from build123d import *

# Parameters (mm, degrees)
BOSS_EXTRUDE1_DEPTH = 115
SKETCH4_W           = 110.804791126
SKETCH4_H           = 80.151186243
CUT_EXTRUDE1_DEPTH  = 15
SKETCH6_W           = 33
SKETCH6_H           = 45.5
CUT_EXTRUDE2_DEPTH  = 40
CUT_EXTRUDE3_DEPTH  = 144.740217058
SKETCH10_W          = 47
SKETCH10_H          = 20
SKETCH10_W_2        = 40
BOSS_EXTRUDE2_DEPTH = 15


with BuildPart() as part:
    # Sketch3 → Boss-Extrude1 (new body)
    with BuildSketch(Plane(origin=(0, 0, 0), x_dir=(0, 0, -1), z_dir=(1, 0, 0))):
        with BuildLine():
            Line((20, -35.767294724), (20, -49.872197862))
            Line((20, -49.872197862), (-20, -49.872197862))
            Line((-20, -49.872197862), (-20, -76.130091706))
            ThreePointArc((-20, -76.130091706), (-55.256322222, -19.163880915), (-10, 30.232705276))
            Line((-10, 30.232705276), (-10, -25.767294724))
            ThreePointArc((-10, -25.767294724), (-7.071067812, -32.838362535), (0, -35.767294724))
            Line((0, -35.767294724), (20, -35.767294724))
        make_face()
    extrude(amount=BOSS_EXTRUDE1_DEPTH)

    # Sketch4 → Cut-Extrude1 (cut)
    with BuildSketch(Plane(origin=(115, 0, 0), x_dir=(0, 0, -1), z_dir=(1, 0, 0))):
        with Locations((-10, -9.842887845)):
            Rectangle(SKETCH4_W, SKETCH4_H)
    extrude(amount=-CUT_EXTRUDE1_DEPTH, mode=Mode.SUBTRACT)

    # Sketch6 → Cut-Extrude2 (cut)
    with BuildSketch(Plane(origin=(0, 31.141039246, 0), x_dir=(1, 0, 0), z_dir=(0, 1, 0))):
        with Locations((46.5, -32.75)):
            Rectangle(SKETCH6_W, SKETCH6_H)
    extrude(amount=-CUT_EXTRUDE2_DEPTH, mode=Mode.SUBTRACT)

    # Sketch9 → Cut-Extrude3 (cut, through all)
    with BuildSketch(Plane(origin=(0, -35.767294724, 0), x_dir=(1, 0, 0), z_dir=(0, 1, 0))):
        with BuildLine():
            Line((90, 5), (10, 5))
            ThreePointArc((10, 5), (5, 10), (10, 15))
            Line((10, 15), (90, 15))
            ThreePointArc((90, 15), (95, 10), (90, 5))
        make_face()
    extrude(amount=-CUT_EXTRUDE3_DEPTH, mode=Mode.SUBTRACT)

    # Sketch10 → Boss-Extrude2 (add)
    with BuildSketch(Plane(origin=(0, 1.141039246, 0), x_dir=(1, 0, 0), z_dir=(0, 1, 0))):
        with Locations((86.5, -15)):
            Rectangle(SKETCH10_W, SKETCH10_H)
        with Locations((10, -15)):
            Rectangle(SKETCH10_W_2, SKETCH10_H)
    extrude(amount=BOSS_EXTRUDE2_DEPTH)


solid = part.part
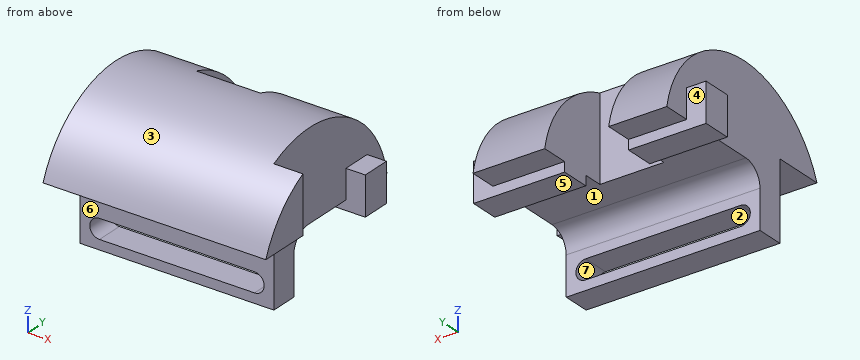
Geometry: final body of the model. Coordinates: model frame, mm. Face numbers are marked on the shaded views. A direction names the side the tool comes from. Give positions to 0.01 mm unless a question says otherwise; leave off trailing zeros. Loops run counter-clockwise (first coordinate to the right, second up) from the corner with the lowest first, then second, coordinate; pieces in that order, holes last. Notation, with made-up numbers: (-1.75, -18.75) - (7.25, -18.75) arc R18 cw to (7.25, 4.25) - close; hole circle Ø1 at (70, 17.5). An arc over 180 degrees is marked (long way). Answer as CSV lines item,"result". Start each with the question number.
1. Section A-A, the plane x = 25. Return loops of the section in (y, z).
2. Section B-B, the plane y = 14. Return loops of the section in (x, z), plus the area to 3 significant figures.
3. Ray query, L1, parallel to X at y = 8, z = 27; L2, parallel to X at y = -20, z = 21.5; L3, parallel to X at y = -51.5, z = 48. Return the intervals inside material, ascending.
4. Section D-D, the plane x = 3.5. Return loops of the section in (y, z).
5. Pin query (flat end, axial travel): P1, Ø10, axis at x = 40.5, z = 36.5, coming from the +Y side; P2, Ø8, axis at x = 30.5, z = 47, coming from the +Y side; P3, Ø4.5, axis at x = 87.5, y = 6.5, coming from the -Z side; P4, Ø1.5, axis at x = 62, y = 13.5, coming from the -Z side. Return the tip coordinate at first contact, or that it passes through.
6. Draft query along Y for the marked faces 1, 2 and 3. Return one class per face: released by +Y, released by -Y, zero draft, split by the parting line, or undercut.
7. Reachability of the marked faces 4, 5, 6 and 7 from +Z, -Z, +X, -X, +Y, -Y: full face, straight path, thin tool, end or side. Return the list, or none.
8. Section C-C, the plane z = -12. Return loops of the section in (x, y).
Answers:
1,outline,"(-76.13, 20) - (-49.87, 20) - (-49.87, -5) - (-35.77, -5) - (-35.77, 0) arc R10 cw to (-25.77, 10) - (1.14, 10) - (1.14, 5) - (16.14, 5) - (16.14, 10) - (30.23, 10) arc R55.5 ccw to start; (-49.87, -20) - (-35.77, -20) - (-35.77, -15) - (-49.87, -15) - close"
2,outline,"(-10, 5) - (30, 5) - (30, 40.11) - (0, 40.11) - (0, 25) - (-10, 25) - close; (63, 5) - (110, 5) - (110, 25) - (100, 25) - (100, 40.11) - (63, 40.11) - close"
2,area,"2,750 mm2"
3,L1,"x = 0 to 30, 63 to 100"
3,L2,"x = 0 to 100"
3,L3,"x = 0 to 115"
4,outline,"(-76.13, 20) - (-49.87, 20) - (-49.87, -20) - (-35.77, -20) - (-35.77, 0) arc R10 cw to (-25.77, 10) - (1.14, 10) - (1.14, 5) - (16.14, 5) - (16.14, 10) - (30.23, 10) arc R55.5 ccw to start"
5,P1,"stops at y = -8.86"
5,P2,"stops at y = 10.69"
5,P3,"stops at z = 5"
5,P4,"passes through"
6,face 1,"undercut"
6,face 2,"zero draft"
6,face 3,"split by the parting line"
7,face 4,"-Z, -X, +Y"
7,face 5,"-Z, +X, -X, +Y"
7,face 6,"-Z, +X, -X, -Y"
7,face 7,"+Y, -Y"
8,outline,"(0, -49.87) - (5.42, -49.87) - (5.42, -35.77) - (0, -35.77) - close; (94.58, -49.87) - (100, -49.87) - (100, -35.77) - (94.58, -35.77) - close"
